Autodesk Inventor part; units mm, degrees
ref_plane "Work Plane1" through (2, 45.282, 44.8195) normal (0, -1, 0) x (1, 0, 0)
ref_plane "YZ Plane" through (0, 0, 0) normal (1, 0, 0) x (0, 1, 0)
ref_plane "XZ Plane" through (0, 0, 0) normal (0, 1, 0) x (-1, 0, 0)
sketch "Sketch1" plane through (0, 0, 0) normal (1, 0, 0) x (0, 1, 0)
  line L0 (7.182, 51.3195) -> (83.382, 51.3195)
  line L1 (83.382, 51.3195) -> (83.382, 13.2195)
  line L2 (83.382, 13.2195) -> (7.182, 13.2195)
  line L3 (7.182, 13.2195) -> (7.182, 51.3195)
  line L4 (39.282, 51.3195) -> (51.282, 51.3195)
  line L5 (51.282, 51.3195) -> (51.282, 44.8195)
  line L6 (51.282, 44.8195) -> (39.282, 44.8195)
  line L7 (39.282, 44.8195) -> (39.282, 51.3195)
  line L8 (45.282, 13.2195) -> (45.282, 51.3195) construction
  line L9 (83.382, 44.8195) -> (65.382, 44.8195)
  line L10 (65.382, 44.8195) -> (65.382, 51.3195)
  line L11 (65.382, 51.3195) -> (83.382, 51.3195)
  line L12 (83.382, 51.3195) -> (83.382, 44.8195)
  line L13 (7.182, 51.3195) -> (25.182, 51.3195)
  line L14 (25.182, 51.3195) -> (25.182, 44.8195)
  line L15 (25.182, 44.8195) -> (7.182, 44.8195)
  line L16 (7.182, 44.8195) -> (7.182, 51.3195)
  circle A0 centre (71.382, 31.3195) radius 3
  circle A1 centre (57.782, 21.3195) radius 3
  circle A2 centre (19.182, 31.3195) radius 3
  circle A3 centre (32.782, 21.3195) radius 3
  point P0 (0, 0)
  point P1 (7.182, 44.8195)
  dimension "d0" = 38.1
  dimension "d1" = 76.2
  dimension "d2" = 12
  dimension "d3" = 6.5
  dimension "d4" = 18
  dimension "d7" = 6
  dimension "d8" = 6
  dimension "d9" = 20
  dimension "d10" = 30
  dimension "d11" = 12.5
  dimension "d12" = 26.1
extrude "Extrusion1" add sketch "Sketch1" along normal blind 2 contours L0 L7 L6 L5 L10 L9 L1 L2 L3 L15 L14
ref_plane "Work Plane1" through (2, 45.282, 44.8195) normal (0, -1, 0) x (1, 0, 0)
sketch "Sketch2" plane through (0, 65.382, 51.3195) normal (0, 1, 0) x (1, 0, 0)
  line L0 (0, 6.5) -> (0, 0)
  line L1 (0, 0) -> (2, 0)
  line L2 (2, 6.5) -> (2, 0)
  line L3 (0, 6.5) -> (2, 6.5)
  circle A0 centre (6, 0) radius 6
  circle A1 centre (6, 0) radius 3.75
  point P0 (0, 51.3195)
  point P1 (2, 4.4721)
  dimension "d13" = 12
  dimension "d14" = 7.5
  dimension "d15" = 4
extrude "Extrusion2" add sketch "Sketch2" against normal up to surface (14.1 mm away) contours L1 L2 A0 picked at (11.1556, -0.7778)
mirror "Mirror1" about plane through (2, 45.282, 44.8195) normal (0, -1, 0) of "Extrusion2"
equation "\"d8\" = d7"
properties part number "zawias-prawy" material "Stainless Steel"
The listing builds one solid part. Answer for the finished solid, in the listing's coordinates (mm). A direction names the side the tool comes from. Give positions to 0.01 mm unless a question says otherwise; leave off trailing zeros. Write each loop counter-clockwise with the first axis right and the second up, starting at its lowest first coordinate (ties: lowest second). Pieces come first, ordered by that corner, then holes. Notation, with made-up numbers: (19.5, 49) - (50.5, 49) arc R22 ccw to (50.5, 63) - close; hole circle Ø6 at (22.25, -30). An arc over 180 degrees is marked (long way). Use a Markdown table: item, result.
1. Find the intervals of material crossed by probe 1 along Z at (x, y) = (6, 61.5); probe 2 along X at (y, z) = (63, 51); probe 3 along Y at (x, z) = (2, 50.5), in increasing order. Write a range as from..to.
Values follow:
| item | result |
|---|---|
| probe 1 | z = 45.32..47.57, 55.07..57.32 |
| probe 2 | x = 0..2.26, 9.74..11.99 |
| probe 3 | y = 25.18..39.28, 51.28..65.38 |
2. Each of these flat-tipped pins is pushed along its axis until it touches: P1, Ø2, axis at x = 0.5, y = 45, coming from the +Z side; P2, Ø3.5, axis at x = 3.5, z = 52, coming from the -Y side; P3, Ø6, axis at x = 8.5, z = 48.5, coming from the +Y side; P4, Ø8, axis at y = 57.78, z = 21.32, coming from the -X side. Where does it stop, or does it pass through?
Values follow:
| item | result |
|---|---|
| P1 | stops at z = 44.82 |
| P2 | stops at y = 25.18 |
| P3 | stops at y = 65.38 |
| P4 | stops at x = 0 |
3. Section B-B on y = 19.5 is taken. Write down the section's boundary in (x, z).
Values follow:
| item | result |
|---|---|
| outline | (0, 13.22) - (2, 13.22) - (2, 28.34) - (0, 28.34) - close; (0, 34.3) - (2, 34.3) - (2, 44.82) - (0, 44.82) - close |
4. Section D-D on y = 36.5 is taken. Write down the section's boundary in (x, z), plus the area to 3 significant figures.
Values follow:
| item | result |
|---|---|
| outline | (0, 13.22) - (2, 13.22) - (2, 46.85) arc R6 ccw (long way) to (0, 51.32) - close; hole circle Ø7.5 at (6, 51.32) |
| area | 139 mm² |
5. Section A-A on x = 6 is taken. Write down the section's boundary in (y, z), plus the area to 3 significant figures.
Values follow:
| item | result |
|---|---|
| outline | (25.18, 45.32) - (39.28, 45.32) - (39.28, 47.57) - (25.18, 47.57) - close; (25.18, 55.07) - (39.28, 55.07) - (39.28, 57.32) - (25.18, 57.32) - close; (51.28, 45.32) - (65.38, 45.32) - (65.38, 47.57) - (51.28, 47.57) - close; (51.28, 55.07) - (65.38, 55.07) - (65.38, 57.32) - (51.28, 57.32) - close |
| area | 127 mm² |
6. Section C-C on x = 10.5 is taken. Write down the section's boundary in (y, z).
Values follow:
| item | result |
|---|---|
| outline | (25.18, 47.35) - (39.28, 47.35) - (39.28, 55.29) - (25.18, 55.29) - close; (51.28, 47.35) - (65.38, 47.35) - (65.38, 55.29) - (51.28, 55.29) - close |
7. For a pull along Z with two mould halves and no side action, classify faces 6 (the cylindrical face through (0.986, 18.532, 34.248)), 7 (the flat face through (1, 75, 44.82)), 8 (the flat face through (2, 39.282, 51)), 9 (the flat face through (1, 46, 13.22)) as released by +Z, released by -Z, zero draft, split by the parting line, or undercut.
Values follow:
| item | result |
|---|---|
| face 6 | undercut |
| face 7 | released by +Z |
| face 8 | zero draft |
| face 9 | released by -Z |
8. A tool of negligible diameter and unlimited length cuts with its end or side. For faces 1 (the cylindrical face through (0.986, 35.553, 22.469)), 2 (the flat face through (1, 16, 44.82)), 3 (the cylindrical face through (5.19, 32.13, 47.66)), 4 (the flat face through (2, 65.382, 51)), 5 (the flat face through (1, 45, 44.82)), from which of +Z, -Z, +X, -X, +Y, -Y can it reach the whole face along a straight path? Write none if from no direction.
Values follow:
| item | result |
|---|---|
| face 1 | +X, -X |
| face 2 | +Z, +X, -X, -Y |
| face 3 | +Y, -Y |
| face 4 | +Z, +X, -X, +Y |
| face 5 | +Z, +X, -X |
